Job drawing, mm, ordinate dimensions from the low corner. One solid piece. Give positions to 0.01 mm unless a question says otherwise; leave off trailing zeros. Loops run counter-clockwise (first coordinate to the right, second up) from the corner with the lowest first, then second, coordinate; pieces in that order, holes last. Notation, with made-up numbers: M 59,24 L 107,24 A18 cw 107,49 Z; hole C 83.25,-36.5 d6. An arc over 180 degrees is marked long. Answer in a Markdown table with one row per item.
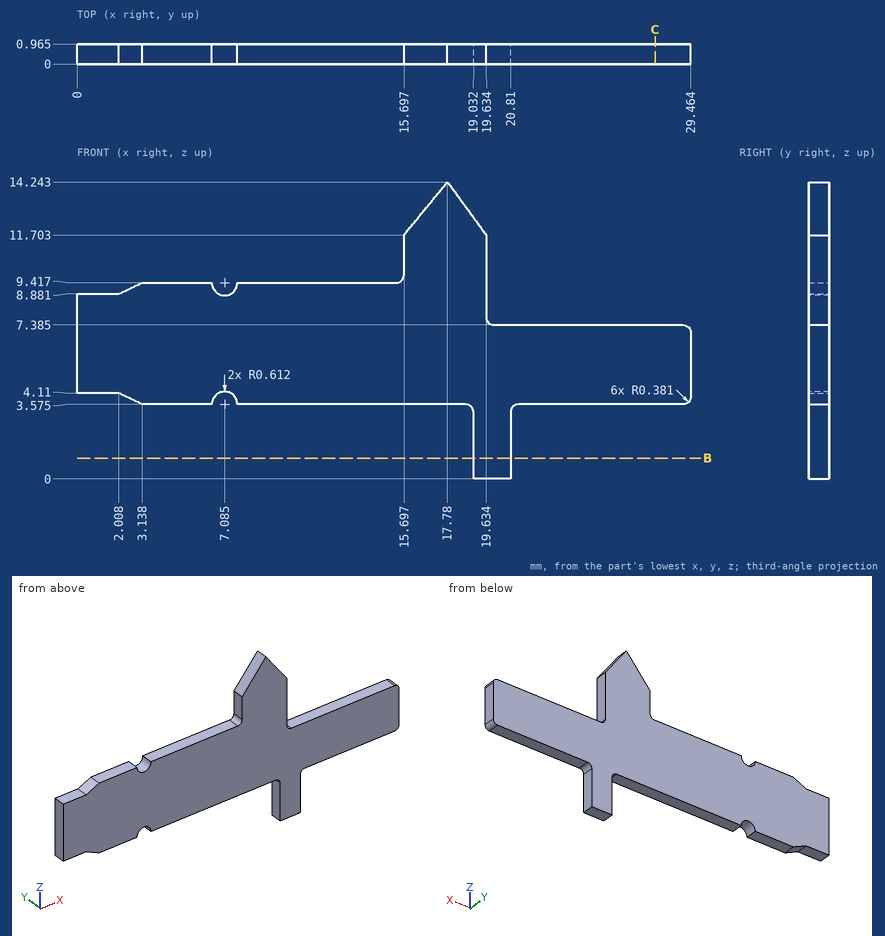
(1) Drill centre lines: line 1 along X through (y, z) = (0.6, 8.5) (1 decimal); line 2 along X through (y, z) = (0.3, 11.5) (1 decimal); line 3 along Z through (x, y) = (9.5, 0.3) (1 decimal). Where is each one in solid material? Low to high.
Recorded:
| item | result |
|---|---|
| line 1 | x = 0 to 19.6 |
| line 2 | x = 15.7 to 19.6 |
| line 3 | z = 3.6 to 9.4 |
(2) Saw through at B-B (z = 1). Write the cut outline in (x, y) (1 decimal).
Recorded:
| item | result |
|---|---|
| outline | M 19,0 L 20.8,0 L 20.8,1 L 19,1 Z |
(3) Saw through at C-C (x = 27.75). Write the cut outline in (y, z) (1 decimal).
Recorded:
| item | result |
|---|---|
| outline | M 0,3.6 L 1,3.6 L 1,7.4 L 0,7.4 Z |
(4) Pin check, flat tips, straight feed: pin 1 Ø5 at (x, z) = (22, 9) entering from -Y; pin 2 Ø0.5 at (x, y) = (4, 0.5) entering from -Z (1 decimal). Stop position of each tip, or through.
Recorded:
| item | result |
|---|---|
| pin 1 | stops at y = 0 |
| pin 2 | stops at z = 3.6 |
